```python
from build123d import *

# Parameters (mm, degrees)
F0_R     = 9.525
F1_DEPTH = 25.4
F2_R     = 11.1125
F3_DEPTH = 7.112
F5_R     = 11.1125
F6_DEPTH = 16.7005
F7_R     = 1.7272
F8_DEPTH = 6.35


with BuildPart() as f1:
    # F0 (on Top) → F1 (new body)
    with BuildSketch(Plane.XY):
        with BuildLine():
            Line((0, 0), (0, -14.2875))
            Line((0, -14.2875), (26.9875, -14.2875))
            Line((26.9875, -14.2875), (26.9875, 0))
            ThreePointArc((26.9875, 0), (13.49375, 13.49375), (0, 0))
        make_face()
        with Locations((13.49375, 0)):
            Circle(F0_R, mode=Mode.SUBTRACT)
    extrude(amount=F1_DEPTH)

    # F2 (on face) → F3 (cut)
    with BuildSketch(Plane.XY.offset(25.4)):
        with Locations((13.49375, 0)):
            Circle(F2_R)
    extrude(amount=-F3_DEPTH, mode=Mode.SUBTRACT)

    # F5 (on face) → F6 (cut, through all)
    with BuildSketch(Plane(origin=(0, 0, 0), x_dir=(1, 0, 0), z_dir=(0, 0, -1))):
        with Locations((13.49375, 0)):
            Circle(F5_R)
    extrude(amount=-F6_DEPTH, mode=Mode.SUBTRACT)

    # F7 (on face) → F8 (cut)
    with BuildSketch(Plane.XZ.offset(14.2875)):
        with Locations((23.01875, 3.96875)):
            Circle(F7_R)
        with Locations((3.96875, 3.96875)):
            Circle(F7_R)
        with Locations((13.49375, 14.31925)):
            Circle(F7_R)
    extrude(amount=-F8_DEPTH, mode=Mode.SUBTRACT)


solid = f1.part
```
Part model, mm, in its own coordinate system. A direction names the side the tool comes from. Coordinates: 2 decimals unless noted, no trailing zeros. Write each loop counter-clockwise with the first axis right and the second up, starting at its lowest first coordinate (ties: lowest second). Pieces come first, ordered by that corner, then holes.
Item 1: Pin check, flat tips, straight feed: pin 1 (8 mm diameter, centred on y = 1, z = 18, fed in from +X); pin 2 (4 mm diameter, centred on x = 23.02, z = 3.97, fed in from +Y); pin 3 (11 mm diameter, centred on x = 8.5, y = -1, fed in from +Z); pin 4 (3 mm diameter, centred on x = 20.5, y = -2.5, fed in from -Z). Stop position of each tip, or through.
Item 2: Slice it at D-D (y = -11.75). Write the cut outline in (x, z).
Item 3: Slice it at C-C (x = 22.5). Write the cut outline in (y, z).
Item 4: Slice it at B-B (x = 14.5). Write the cut outline in (y, z), and give its area (3 significant figures).
Item 5: Mould opens along Y. For faces 5 (the face through (3.98, 0.42, 17.48)), 6 (the face through (13, -14.288, 10)), 7 (the face through (14.422, -12.654, 15.776)) say: released by +Y, released by -Y, zero draft, split by the parting line, or undercut.
Item 6: Probe line 1 (Y direction, x = 13.75, z = 20.5); line 2 (Y direction, x = 11.5, z = 20.5); line 3 (X direction, y = 9.5, z = 9.75). List the from-to ranges inside material, lowest first.
Item 7: Which spindle directions (+Z, -Z, +X, -X, +Y, -Y) get a long thin tool onto all of the face, cutting with end or side? Do faces 1 (the face through (22, 5, 18.288)), 2 (the face through (4, -7.938, 4)), 3 (the face through (0, -7, 13)), 4 (the face through (22, -5, 16.7)). Say none if no direction does.
Results found:
1. pin 1: stops at x = 26.99
1. pin 2: stops at y = 11.2
1. pin 3: stops at z = 18.29
1. pin 4: passes through
2. outline: (0, 0) - (26.99, 0) - (26.99, 25.4) - (0, 25.4) - close; hole circle Ø3.45 at (3.97, 3.97); hole circle Ø3.45 at (13.49, 14.32); hole circle Ø3.45 at (23.02, 3.97)
3. outline: (-14.29, 0) - (-6.51, 0) - (-6.51, 16.7) - (-3.1, 16.7) - (-3.1, 18.29) - (-6.51, 18.29) - (-6.51, 25.4) - (-14.29, 25.4) - (-14.29, 5.62) - (-7.94, 5.62) - (-7.94, 2.32) - (-14.29, 2.32) - close; (3.1, 16.7) - (6.51, 16.7) - (6.51, 0) - (10.05, 0) - (10.05, 25.4) - (6.51, 25.4) - (6.51, 18.29) - (3.1, 18.29) - close
4. outline: (-14.29, 0) - (-11.07, 0) - (-11.07, 12.92) - (-14.29, 12.92) - close; (-14.29, 15.72) - (-11.07, 15.72) - (-11.07, 16.7) - (-9.47, 16.7) - (-9.47, 18.29) - (-11.07, 18.29) - (-11.07, 25.4) - (-14.29, 25.4) - close; (9.47, 16.7) - (11.07, 16.7) - (11.07, 0) - (13.46, 0) - (13.46, 25.4) - (11.07, 25.4) - (11.07, 18.29) - (9.47, 18.29) - close
4. area: 139 mm2
5. face 5: undercut
5. face 6: released by -Y
5. face 7: zero draft
6. line 1: y = -14.29 to -11.11, 11.11 to 13.49
6. line 2: y = -14.29 to -10.93, 10.93 to 13.35
6. line 3: x = 3.91 to 7.73, 19.26 to 23.08
7. face 1: +Z
7. face 2: -Y
7. face 3: +Z, -Z, -X, +Y, -Y
7. face 4: -Z
